```python
from build123d import *

# Parameters (mm, degrees)
SKETCH1_W                   = 35.56
SKETCH1_H                   = 50.8
BOSS_EXTRUDE1_DEPTH         = 10.16
SKETCH2_W                   = 25.4
SKETCH2_H                   = 45.72
CUT_EXTRUDE2_DEPTH          = 5.08
F_40_0_098_DIAMETER_HOLE1_D = 2.4892
SKETCH7_W                   = 23
SKETCH7_H                   = 23
BOSS_EXTRUDE2_DEPTH         = 30
FILLET1_R                   = 1.778
CUT_EXTRUDE3_DEPTH          = 74.878137497


with BuildPart() as part:
    # Sketch1 → Boss-Extrude1 (new body)
    with BuildSketch(Plane.XY):
        with Locations((-17.78, 25.4)):
            Rectangle(SKETCH1_W, SKETCH1_H)
    extrude(amount=BOSS_EXTRUDE1_DEPTH)

    # Sketch2 → Cut-Extrude2 (cut)
    with BuildSketch(Plane.XY.offset(10.16)):
        with Locations((-17.792594088, 27.94)):
            Rectangle(SKETCH2_W, SKETCH2_H)
    extrude(amount=-CUT_EXTRUDE2_DEPTH, mode=Mode.SUBTRACT)

    # #40 (0.098) Diameter Hole1 (through all)
    with Locations(Plane(origin=(0, 0, 0), x_dir=(-1, 0, 0), z_dir=(0, 0, -1))):
        with Locations((2.792369004, 43.087106138), (2.792369004, 26.092979092), (2.792369004, 9.105182099), (9.290740849, 2.822744672), (26.292369004, 2.787106138), (32.780032006, 9.105182099), (32.792369004, 26.087106138), (32.792369004, 43.087106138)):
            Hole(F_40_0_098_DIAMETER_HOLE1_D / 2)

    # Sketch7 → Boss-Extrude2 (add)
    with BuildSketch(Plane(origin=(0, 0, 0), x_dir=(-1, 0, 0), z_dir=(0, 0, -1))):
        with Locations((17.947498481, 29.656487967)):
            Rectangle(SKETCH7_W, SKETCH7_H)
        Polygon((15.026504795, 33.68344643), (21.026504795, 33.68344643), (24.026504795, 36.68344643), (24.026504795, 37.68344643), (21.026504795, 37.68344643), (21.026504795, 39.757316979), (28.107693687, 39.757316979), (28.107693687, 32.595354636), (26.021869747, 32.595354636), (26.026504795, 35.68344643), (25.026504795, 35.68344643), (22.026504795, 32.68344643), (22.026504795, 26.68344643), (25.026504795, 23.68344643), (26.026504795, 23.68344643), (26.026504795, 26.68344643), (28.026504795, 26.68344643), (28.026504795, 19.631136525), (21.026504795, 19.68344643), (21.026504795, 21.68344643), (24.026504795, 21.68344643), (24.026504795, 22.68344643), (21.026504795, 25.68344643), (15.026504795, 25.68344643), (12.026504795, 22.68344643), (12.026504795, 21.68344643), (15.026504795, 21.68344643), (15.026504795, 19.68344643), (7.971438759, 19.68344643), (8.026504795, 26.68344643), (10.026504795, 26.68344643), (10.026504795, 23.68344643), (11.026504795, 23.68344643), (14.026504795, 26.68344643), (14.026504795, 32.68344643), (11.026504795, 35.68344643), (10.026504795, 35.68344643), (10.026504795, 32.68344643), (8.026504795, 32.68344643), (8.026504795, 39.757316979), (15.097897728, 39.757316979), (15.026504795, 37.68344643), (12.026504795, 37.68344643), (12.026504795, 36.68344643), align=None, mode=Mode.SUBTRACT)
    extrude(amount=BOSS_EXTRUDE2_DEPTH)

    # Fillet1
    fillet1_edges = [part.edges().sort_by_distance(p)[0] for p in [
        (-6.447498481, 29.656487967, 0),
        (-17.947498481, 18.156487967, 0),
        (-29.447498481, 29.656487967, 0),
        (-17.947498481, 41.156487967, 0),
    ]]
    fillet(fillet1_edges, radius=FILLET1_R)

    # Sketch8 → Cut-Extrude3 (cut, through all)
    with BuildSketch(Plane.XY.offset(10.16)):
        Polygon((-5.178964387, 50.8), (0, 44.392134486), (0, 50.8), align=None)
        Polygon((-35.56, 44.706622517), (-35.56, 50.8), (-30.402645731, 50.8), align=None)
        Polygon((-35.56, 5.970049098), (-35.56, 0), (-30.492594088, 0), align=None)
        Polygon((-5.092594088, -0.031324356), (0, 0), (0, 5.970049098), align=None)
    extrude(amount=-CUT_EXTRUDE3_DEPTH, mode=Mode.SUBTRACT)


solid = part.part
```
Geometry check sheet. Reference: the model listing, model coordinates, mm. A direction names the side the tool comes from. Give positions to 0.01 mm unless a question says otherwise; leave off trailing zeros. Order: outer loops, then holes, each group sorted by start corner. A loop starts at its lowest first (then second) coordinate and runs counter-clockwise, first axis right, second up. Notation, with made-up numbers: (12.25, -1.5) - (69.25, -1.5) arc R25 ccw to (69.25, 30.5) - close; hole circle Ø9 at (78.5, -32). An arc over 180 degrees is marked (long way). Answer in a Markdown table with one row per item. Add a question column.
Q1. Cross-section at D-D, the plane y = 32. Enter the section's corners in (x, z), then the cut area to 3 significant figures.
Q2. Mould release check, pull along Y, two halves, no side actions. Record for faces 3 (the flat face through (-30.493, 28, 8)), 4 (the flat face through (-18, 5.08, 8)), 5 (the cylindrical face through (-27.536, 2.842, 5.151)): pulls with the +Y half, pulls with the -Y half, needs draft (parallel to the pull), parting line crosses it, or undercut.
Q3. Cross-section at B-B, the plane z = 7.5. Count the separate pieces of the cut face and the enclosed holes in it, then the cut area to 3 significant figures.
Q4. Tool access check on faces 1 (the flat face through (0, 25, 5)), 2 (the flat face through (-28.027, 23, -15)). Record the directions out of +Z, -Z, +X, -X, +Y, -Y that give a thin tool (end or side, any length) a straight path to the whole face; none if there is none.
Q5. Material ranges on probe 1 along X at (y, z) = (20.5, -3); probe 2 along Y at (x, z) = (-16.5, -3); probe 3 along Y at (x, z) = (-14.5, -18.5), recorded low to high. Write a range as from..to.
Q6. Cross-section at C-C, the plane y = 8.5. Enter the section's corners in (x, z), then the cut area to 3 significant figures.
Q7. Cross-section at A-A, the plane x = -20. Enter the section's corners in (y, z), then the cut area to 3 significant figures.
Q8. Gauge pin test, flat ends, axial feed: pin 1 (1.1 mm diameter, centred on y = 37.5, z = -17.5, fed in from -X); pin 2 (8 mm diameter, centred on x = -20.5, z = -19.5, fed in from +Y); pin 3 (1 mm diameter, centred on x = -27, z = -12, fed in from -Y); pin 4 (2 mm diameter, centred on x = -32.79, y = 43.09, fed in from -Z). Record the tip position at first contact, or that the pin passes through.
Check values:
| question | item | result |
|---|---|---|
| 1 | outline | (-35.56, 0) - (-31.23, 0) arc R1.78 cw to (-29.45, -1.78) - (-29.45, -30) - (-22.03, -30) - (-22.03, 0) - (-14.03, 0) - (-14.03, -30) - (-6.45, -30) - (-6.45, -1.78) arc R1.78 cw to (-4.67, 0) - (0, 0) - (0, 10.16) - (-5.09, 10.16) - (-5.09, 5.08) - (-30.49, 5.08) - (-30.49, 10.16) - (-35.56, 10.16) - close |
| 1 | area | 684 mm^2 |
| 2 | face 3 | needs draft |
| 2 | face 4 | pulls with the +Y half |
| 2 | face 5 | undercut |
| 3 | separate pieces | 1 |
| 3 | enclosed holes | 8 |
| 3 | area | 544 mm^2 |
| 4 | face 1 | +Z, -Z, +X, +Y, -Y |
| 4 | face 2 | -Z |
| 5 | probe 1 | x = -29.45..-28.03, -21.03..-15.03, -7.98..-6.45 |
| 5 | probe 2 | y = 18.16..25.68, 33.68..41.16 |
| 5 | probe 3 | y = 18.16..19.68, 21.68..25.16, 34.21..37.68, 39.76..41.16 |
| 6 | outline | (-35.56, 0) - (-33.87, 0) - (-33.87, 10.16) - (-35.56, 10.16) - close; (-31.69, 0) - (-3.88, 0) - (-3.88, 10.16) - (-5.09, 10.16) - (-5.09, 5.08) - (-30.49, 5.08) - (-30.49, 10.16) - (-31.69, 10.16) - close; (-1.7, 0) - (0, 0) - (0, 10.16) - (-1.7, 10.16) - close |
| 6 | area | 188 mm^2 |
| 7 | outline | (0, 0) - (16.38, 0) arc R1.78 cw to (18.16, -1.78) - (18.16, -30) - (25.68, -30) - (25.68, 0) - (33.68, 0) - (33.68, -30) - (41.16, -30) - (41.16, -1.78) arc R1.78 cw to (42.93, 0) - (50.8, 0) - (50.8, 5.08) - (5.08, 5.08) - (5.08, 10.16) - (0, 10.16) - close |
| 7 | area | 735 mm^2 |
| 8 | pin 1 | stops at x = -29.45 |
| 8 | pin 2 | stops at y = 41.16 |
| 8 | pin 3 | stops at y = 18.16 |
| 8 | pin 4 | passes through |
